Build history of the part. All positions in model axes, mm. Face numbers are marked on the shaded views. A direction names the side the tool comes from. Give positions to 0.01 mm unless a question says otherwise; leave off trailing zeros. Order: outer loops, then holes, each group sorted by start corner. A loop starts at its lowest first (then second) coordinate and runs counter-clockwise, first axis right, second up. Notation, with made-up numbers: M 86.25,-10.5 L 137.25,-10.5 A20 cw 137.25,9.5 Z; hole C 72,-19.5 d8. An arc over 180 degrees is marked long. Use CSV: the item, a comma, the result in double quotes. Start each with the question number.
Item 1: Band-saw the part on C-C on z = -7.62. Write the cut outline in (x, y), plus the area to 3 significant figures.
Item 2: Band-saw the part on A-A on y = -8. Write the cut outline in (x, z) (1 decimal), plus the area to 3 significant figures.
Item 3: Pin check, flat tips, straight feed: P1, Ø12, axis at x = 18, z = 7, coming from the +Y side (3 decimals); P2, Ø2, axis at x = -35, y = -10.5, coming from the -Z side; P3, Ø7.5, axis at x = 31.75, z = 43.18, coming from the -Y side; P4, Ø10.5, axis at y = -13.5, z = 30.5, coming from the -X side. Stop position of each tip, or through.
Item 4: Wall check: line 1 along X through (y, z) = (-20.1, 43.18); line 2 along Z through (x, y) = (-5, -11) (3 decimals); line 3 along Y through (x, z) = (-17, 26). Give the ranges that are in metal, low to high.
Item 5: Band-saw the part on B-B on x = 6. Write the cut outline in (y, z) (3 decimals).
Item 6: Band-saw the part on D-D on z = 5.5. Write the cut outline in (x, y) (1 decimal), plus the area to 3 significant figures.
Item 7: Two-plate mould, pull along Z, no slides. Class the marked faces 1, 2 and 3: pulls with the +Z half, pulls with the -Z half, needs draft (parallel to the pull), parting line crosses it, or undercut.
Item 8: Which spindle directions (+Z, -Z, +X, -X, +Y, -Y) get a long thin tool onto all of the face, cutting with end or side? Do the marked faces 4, 5, 6, 7 and 8. Say none if no direction does.
from build123d import *

# Parameters (mm, degrees)
SKETCH1_W            = 76.2
SKETCH1_H            = 35.56
BOSS_EXTRUDE1_DEPTH  = 1.905
SKETCH2_R            = 2.38125
CUT_EXTRUDE1_DEPTH   = 6.35
SKETCH3_W            = 41.402
SKETCH3_H            = 21.59
CUT_EXTRUDE2_DEPTH   = 3.81
SKETCH5_W            = 76.2
SKETCH5_H            = 76.2
BOSS_EXTRUDE2_DEPTH  = 3.81
SKETCH8_R            = 2.667
CUT_EXTRUDE5_DEPTH   = 3.81
BOSS_EXTRUDE4_START  = 6.096
SKETCH9_R            = 4.445
SKETCH9_R_2          = 2.667
BOSS_EXTRUDE4_DEPTH  = 6.096
SKETCH10_W           = 6.985
SKETCH10_H           = 18.205369343
BOSS_EXTRUDE5_DEPTH  = 6.096
SKETCH11_R           = 4.445
SKETCH11_R_2         = 2.667
BOSS_EXTRUDE6_DEPTH  = 5.08
SKETCH12_W           = 6.985
SKETCH12_H           = 18.205369343
BOSS_EXTRUDE7_DEPTH  = 5.08
SKETCH13_R           = 2.3495
CUT_EXTRUDE6_DEPTH   = 72.898153662
BOSS_EXTRUDE8_START  = 15.466000132
SKETCH14_R           = 2.38125
SKETCH14_R_2         = 2.667
SKETCH14_W           = 41.402
SKETCH14_H           = 21.59
BOSS_EXTRUDE8_DEPTH  = 15.466000132
CUT_EXTRUDE7_START   = -15.39000003
SKETCH15_R           = 2.38125
SKETCH15_W           = 41.402
SKETCH15_H           = 21.59
CUT_EXTRUDE7_DEPTH   = 15.39000003
CUT_EXTRUDE8_START   = -8.001
SKETCH16_R           = 2.667
CUT_EXTRUDE8_DEPTH   = 8.001
FILLET1_R            = 2.54
CHAMFER1_SIZE        = 3.81
FILLET2_R            = 8.89
SKETCH17_W           = 5.08
SKETCH17_H           = 25.4
BOSS_EXTRUDE9_DEPTH  = 76.2
SKETCH18_W           = 38.1
SKETCH18_H           = 15.24
SKETCH18_W_2         = 35.56
SKETCH18_H_2         = 12.7
BOSS_EXTRUDE10_DEPTH = 11.43
CHAMFER2_SIZE        = 1.905
FILLET3_R            = 2.54
SKETCH19_R           = 2.3495
CUT_EXTRUDE9_DEPTH   = 8.89
SKETCH20_W           = 6.985
SKETCH20_H           = 16.51
CUT_EXTRUDE10_DEPTH  = 1.27
FILLET4_R            = 2.54


with BuildPart() as part:
    # Sketch1 → Boss-Extrude1 (new, symmetric)
    with BuildSketch(Plane.XY):
        Rectangle(SKETCH1_W, SKETCH1_H)
    extrude(amount=BOSS_EXTRUDE1_DEPTH, both=True)

    # Sketch2 → Cut-Extrude1 (cut)
    with BuildSketch(Plane.XY.offset(1.905)):
        with Locations((-18.034, 8.734933)):
            Circle(SKETCH2_R)
        with Locations((30.734, 8.734933)):
            Circle(SKETCH2_R)
        with Locations((30.734, -1.114933)):
            Circle(SKETCH2_R)
        with Locations((-18.034, -1.114933)):
            Circle(SKETCH2_R)
    extrude(amount=-CUT_EXTRUDE1_DEPTH, mode=Mode.SUBTRACT)

    # Sketch3 → Cut-Extrude2 (cut)
    with BuildSketch(Plane.XY.offset(1.905)):
        with Locations((6.35, 3.81)):
            Rectangle(SKETCH3_W, SKETCH3_H)
    extrude(amount=-CUT_EXTRUDE2_DEPTH, mode=Mode.SUBTRACT)

    # Sketch5 → Boss-Extrude2 (add)
    with BuildSketch(Plane.XZ.offset(17.78)):
        with Locations((0, 11.43)):
            Rectangle(SKETCH5_W, SKETCH5_H)
    extrude(amount=BOSS_EXTRUDE2_DEPTH)

    # Sketch8 → Cut-Extrude5 (cut)
    with BuildSketch(Plane(origin=(0, 0, -1.905), x_dir=(-1, 0, 0), z_dir=(0, 0, -1))):
        with Locations((33.528, 3.175)):
            Circle(SKETCH8_R)
    extrude(amount=-CUT_EXTRUDE5_DEPTH, mode=Mode.SUBTRACT)

    # Sketch9 → Boss-Extrude4 (add)
    with BuildSketch(Plane(origin=(0, 0, -1.905), x_dir=(-1, 0, 0), z_dir=(0, 0, -1)).offset(BOSS_EXTRUDE4_START)):
        with Locations(Location((33.528, 3.175, 0), (0, 0, 180))):
            Circle(SKETCH9_R)
        with Locations((33.528, 3.175)):
            Circle(SKETCH9_R_2, mode=Mode.SUBTRACT)
    extrude(amount=-BOSS_EXTRUDE4_DEPTH)

    # Sketch10 → Boss-Extrude5 (add)
    with BuildSketch(Plane(origin=(0, 0, -1.905), x_dir=(-1, 0, 0), z_dir=(0, 0, -1))):
        with Locations((33.528, -8.677315329)):
            Rectangle(SKETCH10_W, SKETCH10_H)
    extrude(amount=BOSS_EXTRUDE5_DEPTH)

    # Sketch11 → Boss-Extrude6 (add)
    with BuildSketch(Plane.XY.offset(1.905)):
        with Locations(Location((-33.528, 3.175, 0), (0, 0, 180))):
            Circle(SKETCH11_R)
        with Locations(Location((-33.528, 3.175, 0), (0, 0, 180))):
            Circle(SKETCH11_R_2, mode=Mode.SUBTRACT)
    extrude(amount=BOSS_EXTRUDE6_DEPTH)

    # Sketch12 → Boss-Extrude7 (add)
    with BuildSketch(Plane.XY.offset(1.905)):
        with Locations((-33.528, -8.677315329)):
            Rectangle(SKETCH12_W, SKETCH12_H)
    extrude(amount=BOSS_EXTRUDE7_DEPTH)

    # Sketch13 → Cut-Extrude6 (cut, through all)
    with BuildSketch(Plane(origin=(0, -17.78, 0), x_dir=(1, 0, 0), z_dir=(0, 1, 0))):
        with Locations(Location((-19.05, 20.32, 0), (0, 0, 90))):
            Circle(SKETCH13_R)
        with Locations(Location((31.75, 20.32, 0), (0, 0, 90))):
            Circle(SKETCH13_R)
        with Locations(Location((31.75, -43.18, 0), (0, 0, 270))):
            Circle(SKETCH13_R)
        with Locations(Location((-19.05, -43.18, 0), (0, 0, 270))):
            Circle(SKETCH13_R)
    extrude(amount=-CUT_EXTRUDE6_DEPTH, mode=Mode.SUBTRACT)

    # Sketch14 → Boss-Extrude8 (add)
    with BuildSketch(Plane.XY.offset(1.905).offset(BOSS_EXTRUDE8_START)):
        Polygon((-30.0355, -17.78), (38.1, -17.78), (38.1, 17.78), (-38.1, 17.78), (-38.1, -17.78), (-37.0205, -17.78), align=None)
        with Locations((30.734, -1.114933)):
            Circle(SKETCH14_R, mode=Mode.SUBTRACT)
        with Locations((30.734, 8.734933)):
            Circle(SKETCH14_R, mode=Mode.SUBTRACT)
        with Locations((-18.034, -1.114933)):
            Circle(SKETCH14_R, mode=Mode.SUBTRACT)
        with Locations((-18.034, 8.734933)):
            Circle(SKETCH14_R, mode=Mode.SUBTRACT)
        with Locations(Location((-33.528, 3.175, 0), (0, 0, 180))):
            Circle(SKETCH14_R_2, mode=Mode.SUBTRACT)
        with Locations((6.35, 3.81)):
            Rectangle(SKETCH14_W, SKETCH14_H, mode=Mode.SUBTRACT)
    extrude(amount=-BOSS_EXTRUDE8_DEPTH)

    # Sketch15 → Cut-Extrude7 (cut)
    with BuildSketch(Plane(origin=(0, 0, -1.905), x_dir=(-1, 0, 0), z_dir=(0, 0, -1)).offset(CUT_EXTRUDE7_START)):
        with BuildLine():
            Line((-38.1, -17.78), (30.0355, -17.78))
            Line((30.0355, -17.78), (30.0355, 0.425369343))
            ThreePointArc((30.0355, 0.425369343), (33.528, 7.62), (37.0205, 0.425369343))
            Line((37.0205, 0.425369343), (37.0205, -17.78))
            Line((37.0205, -17.78), (38.1, -17.78))
            Line((38.1, -17.78), (38.1, 17.78))
            Line((38.1, 17.78), (-38.1, 17.78))
            Line((-38.1, 17.78), (-38.1, -17.78))
        make_face()
        with Locations(Location((18.034, -1.114933, 0), (0, 0, 180))):
            Circle(SKETCH15_R, mode=Mode.SUBTRACT)
        with Locations(Location((18.034, 8.734933, 0), (0, 0, 180))):
            Circle(SKETCH15_R, mode=Mode.SUBTRACT)
        with Locations(Location((-30.734, -1.114933, 0), (0, 0, 180))):
            Circle(SKETCH15_R, mode=Mode.SUBTRACT)
        with Locations(Location((-30.734, 8.734933, 0), (0, 0, 180))):
            Circle(SKETCH15_R, mode=Mode.SUBTRACT)
        with Locations((-6.35, 3.81)):
            Rectangle(SKETCH15_W, SKETCH15_H, mode=Mode.SUBTRACT)
    extrude(amount=CUT_EXTRUDE7_DEPTH, mode=Mode.SUBTRACT)

    # Sketch16 → Cut-Extrude8 (cut)
    with BuildSketch(Plane(origin=(0, 0, -8.001), x_dir=(-1, 0, 0), z_dir=(0, 0, -1)).offset(CUT_EXTRUDE8_START)):
        with BuildLine():
            Line((30.0355, 0.425369343), (30.0355, -17.78))
            Line((30.0355, -17.78), (37.0205, -17.78))
            Line((37.0205, -17.78), (37.0205, 0.425369343))
            ThreePointArc((37.0205, 0.425369343), (33.528, 7.62), (30.0355, 0.425369343))
        make_face()
        with Locations((33.528, 3.175)):
            Circle(SKETCH16_R, mode=Mode.SUBTRACT)
    extrude(amount=CUT_EXTRUDE8_DEPTH, mode=Mode.SUBTRACT)

    # Fillet1
    fillet1_edges = [part.edges().sort_by_distance(p)[0] for p in [
        (38.1, -19.685, -26.67),
        (38.1, -19.685, 49.53),
        (-38.1, -19.685, 49.53),
        (-38.1, -19.685, -26.67),
    ]]
    fillet(fillet1_edges, radius=FILLET1_R)

    # Chamfer1
    chamfer1_edges = [part.edges().sort_by_distance(p)[0] for p in [
        (0, -17.78, 17.371000132),
        (4.03225, -17.78, 13.48500003),
    ]]
    chamfer(chamfer1_edges, length=CHAMFER1_SIZE)

    # Fillet2
    fillet2_edges = [part.edges().sort_by_distance(p)[0] for p in [
        (-38.1, 17.78, 15.428000081),
    ]]
    fillet(fillet2_edges, radius=FILLET2_R)

    # Sketch17 → Boss-Extrude9 (add)
    with BuildSketch(Plane(origin=(0, 0, -26.67), x_dir=(-1, 0, 0), z_dir=(0, 0, -1))):
        with Locations((35.56, -34.29)):
            Rectangle(SKETCH17_W, SKETCH17_H)
    extrude(amount=-BOSS_EXTRUDE9_DEPTH)

    # Sketch18 → Boss-Extrude10 (add)
    with BuildSketch(Plane(origin=(0, -17.78, 0), x_dir=(1, 0, 0), z_dir=(0, 1, 0))):
        with Locations((6.35, -31.976000132)):
            Rectangle(SKETCH18_W, SKETCH18_H)
        with Locations((6.35, -31.976000132)):
            Rectangle(SKETCH18_W_2, SKETCH18_H_2, mode=Mode.SUBTRACT)
    extrude(amount=BOSS_EXTRUDE10_DEPTH)

    # Chamfer2
    chamfer2_edges = [part.edges().sort_by_distance(p)[0] for p in [
        (6.35, -17.78, 25.626000132),
        (24.13, -17.78, 31.976000132),
        (-12.7, -17.78, 31.976000132),
        (6.35, -17.78, 39.596000132),
        (25.4, -17.78, 31.976000132),
        (6.35, -17.78, 24.356000132),
        (-11.43, -17.78, 31.976000132),
        (6.35, -17.78, 38.326000132),
    ]]
    chamfer(chamfer2_edges, length=CHAMFER2_SIZE)

    # Fillet3
    fillet3_edges = [part.edges().sort_by_distance(p)[0] for p in [
        (-38.1, -34.29, 49.53),
        (-38.1, -34.29, -26.67),
    ]]
    fillet(fillet3_edges, radius=FILLET3_R)

    # Sketch19 → Cut-Extrude9 (cut)
    with BuildSketch(Plane.ZY.offset(38.1)):
        with Locations((-7.62, -32.385)):
            Circle(SKETCH19_R)
        with Locations(Location((30.48, -32.385, 0), (0, 0, 180))):
            Circle(SKETCH19_R)
    extrude(amount=-CUT_EXTRUDE9_DEPTH, mode=Mode.SUBTRACT)

    # Sketch20 → Cut-Extrude10 (cut)
    with BuildSketch(Plane(origin=(0, 0, 0), x_dir=(-1, 0, 0), z_dir=(0, 0, -1))):
        with Locations((33.528, -9.525)):
            Rectangle(SKETCH20_W, SKETCH20_H)
    extrude(amount=-CUT_EXTRUDE10_DEPTH, mode=Mode.SUBTRACT)

    # Fillet4
    # the kernel refuses this fillet: 2.54 mm, written as the material it adds along each edge
    with BuildSketch(Plane(origin=(-37.0205, -1.27, 1.27), x_dir=(0, -1, 0), z_dir=(1, 0, 0))) as fillet4_piece_1:
        with BuildLine():
            CenterArc((2.199704526, 2.54), FILLET4_R, 210, 60)
            Line((0, 1.27), (-0.043994091, 1.2446))
            ThreePointArc((-0.043994091, 1.2446), (-0.0508, 0.635), (-0.0508, 0))
            Line((-0.0508, 0), (0, -0.0508))
            Line((0, -0.0508), (2.199704526, -0.0508))
            Line((2.199704526, -0.0508), (2.199704526, 0))
        make_face()
    extrude(amount=6.985)


solid = part.part
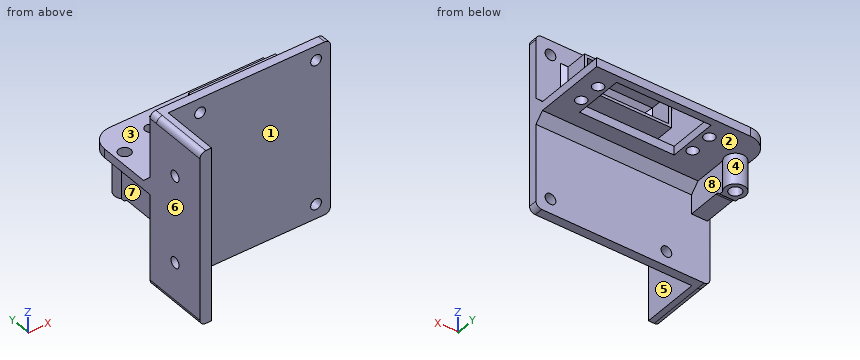
Model answer:
1,outline,"M -38.1,-46.99 L -33.02,-46.99 L -33.02,-34.73 L -38.1,-34.73 Z; M -38.1,-30.04 L -33.02,-30.04 L -33.02,-21.59 L 38.1,-21.59 L 38.1,-17.78 L -38.1,-17.78 Z"
1,area,"395 mm^2"
2,outline,"M -38.1,13.5 L -37,13.5 L -37,1.3 L -30,1.3 L -30,13.5 L 38.1,13.5 L 38.1,17.4 L -38.1,17.4 Z; M -12.7,24.4 L 25.4,24.4 L 25.4,39.6 L -12.7,39.6 Z; hole M -11.4,25.6 L 24.1,25.6 L 24.1,38.3 L -11.4,38.3 Z"
2,area,"510 mm^2"
3,P1,"stops at y = -14.455"
3,P2,"stops at z = 1.27"
3,P3,"stops at y = -21.59"
3,P4,"stops at x = -38.1"
4,line 1,"x = -38.1 to -21.4, -16.7 to 29.4, 34.1 to 38.1"
4,line 2,"z = 13.485 to 17.371, 24.356 to 25.626, 38.326 to 39.596"
4,line 3,"y = -21.59 to -17.78"
5,outline,"M -21.59,-26.67 L -17.78,-26.67 L -17.78,9.675 L -13.97,13.485 L -6.985,13.485 L -6.985,17.371 L -13.97,17.371 L -17.78,21.181 L -17.78,22.451 L -15.875,24.356 L -6.35,24.356 L -6.35,25.626 L -15.875,25.626 L -17.78,27.531 L -17.78,36.421 L -15.875,38.326 L -6.35,38.326 L -6.35,39.596 L -15.875,39.596 L -17.78,41.501 L -17.78,49.53 L -21.59,49.53 Z; M 14.605,13.485 L 17.78,13.485 L 17.78,17.371 L 14.605,17.371 Z"
6,outline,"M -38.1,-47 L -33,-47 L -33,-21.6 L 38.1,-21.6 L 38.1,-17.8 L -30,-17.8 L -30,0.4 A4.4 ccw long -37,0.4 L -37,-17.8 L -38.1,-17.8 Z; hole C -33.5,3.2 d5.3"
6,area,"578 mm^2"
7,face 1,"needs draft"
7,face 2,"pulls with the -Z half"
7,face 3,"undercut"
8,face 4,"-Z"
8,face 5,"+Z, -Z, +X, -Y"
8,face 6,"+Z, -Z, -X, +Y, -Y"
8,face 7,"-Z, -X"
8,face 8,"-Z, +X"
